from build123d import *

# Parameters (mm, degrees)
BOSS_EXTRUDE1_DEPTH = 5
SKETCH4_R           = 2.5
CUT_EXTRUDE1_DEPTH  = 20
CUT_EXTRUDE2_DEPTH  = 10
SKETCH8_R           = 2.5
CUT_EXTRUDE3_DEPTH  = 10


with BuildPart() as part:
    # Sketch1 → Boss-Extrude1 (new body)
    with BuildSketch(Plane(origin=(0, 0, 0), x_dir=(1, 0, 0), z_dir=(0, 1, 0))):
        with BuildLine():
            Line((-279.827757823, 163.191662052), (-273.826637764, 163.191662052))
            ThreePointArc((-273.826637764, 163.191662052), (-271.35176403, 162.166535786), (-270.326637764, 159.691662052))
            Line((-270.326637764, 159.691662052), (-270.326637764, 137.406790352))
            Line((-270.326637764, 137.406790352), (-275.326637764, 137.406790352))
            Line((-275.326637764, 137.406790352), (-275.326637764, -155.644744292))
            Line((-275.326637764, -155.644744292), (-270.326637764, -155.644744292))
            Line((-270.326637764, -155.644744292), (-270.326637764, -177.929615992))
            ThreePointArc((-270.326637764, -177.929615992), (-271.35176403, -180.404489727), (-273.826637764, -181.429615992))
            Line((-273.826637764, -181.429615992), (-279.827757823, -181.429615992))
            ThreePointArc((-279.827757823, -181.429615992), (-293.34742446, -188.470830973), (-295.328317853, -203.584935503))
            ThreePointArc((-295.328317853, -203.584935503), (-279.434102169, -225.521844766), (-254.372898367, -235.807278357))
            ThreePointArc((-254.372898367, -235.807278357), (-245.944078079, -233.964230965), (-239.597831877, -228.11897697))
            Line((-239.597831877, -228.11897697), (-235.326637764, -228.11897697))
            Line((-235.326637764, -228.11897697), (-235.326637764, -233.11897697))
            Line((-235.326637764, -233.11897697), (161.673362236, -233.11897697))
            Line((161.673362236, -233.11897697), (161.673362236, -228.11897697))
            Line((161.673362236, -228.11897697), (165.944556349, -228.11897697))
            ThreePointArc((165.944556349, -228.11897697), (172.290802551, -233.964230965), (180.719622838, -235.807278357))
            ThreePointArc((180.719622838, -235.807278357), (205.780826641, -225.521844766), (221.675042324, -203.584935503))
            ThreePointArc((221.675042324, -203.584935503), (219.694148932, -188.470830973), (206.174482295, -181.429615992))
            Line((206.174482295, -181.429615992), (200.173362236, -181.429615992))
            ThreePointArc((200.173362236, -181.429615992), (197.698488502, -180.404489727), (196.673362236, -177.929615992))
            Line((196.673362236, -177.929615992), (196.673362236, -155.644744292))
            Line((196.673362236, -155.644744292), (201.673362236, -155.644744292))
            Line((201.673362236, -155.644744292), (201.673362236, 137.406790352))
            Line((201.673362236, 137.406790352), (196.673362236, 137.406790352))
            Line((196.673362236, 137.406790352), (196.673362236, 159.691662052))
            ThreePointArc((196.673362236, 159.691662052), (197.698488502, 162.166535786), (200.173362236, 163.191662052))
            Line((200.173362236, 163.191662052), (206.174482295, 163.191662052))
            ThreePointArc((206.174482295, 163.191662052), (219.694148932, 170.232877033), (221.675042324, 185.346981563))
            ThreePointArc((221.675042324, 185.346981563), (205.780826641, 207.283890825), (180.719622838, 217.569324417))
            ThreePointArc((180.719622838, 217.569324417), (172.290802551, 215.726277025), (165.944556349, 209.88102303))
            Line((165.944556349, 209.88102303), (161.673362236, 209.88102303))
            Line((161.673362236, 209.88102303), (161.673362236, 214.88102303))
            Line((161.673362236, 214.88102303), (-235.326637764, 214.88102303))
            Line((-235.326637764, 214.88102303), (-235.326637764, 209.88102303))
            Line((-235.326637764, 209.88102303), (-239.597831877, 209.88102303))
            ThreePointArc((-239.597831877, 209.88102303), (-245.944078079, 215.726277025), (-254.372898367, 217.569324417))
            ThreePointArc((-254.372898367, 217.569324417), (-279.434102169, 207.283890825), (-295.328317853, 185.346981563))
            ThreePointArc((-295.328317853, 185.346981563), (-293.34742446, 170.232877033), (-279.827757823, 163.191662052))
        make_face()
    extrude(amount=BOSS_EXTRUDE1_DEPTH)

    # Sketch4 → Cut-Extrude1 (cut)
    with BuildSketch(Plane.XZ):
        with Locations(Location((-201.826637764, 124.11897697, 0), (0, 0, 270))):
            Circle(SKETCH4_R)
        with Locations(Location((-201.826637764, -105.88102303, 0), (0, 0, 90))):
            Circle(SKETCH4_R)
        with Locations(Location((128.173362236, -105.88102303, 0), (0, 0, 270))):
            Circle(SKETCH4_R)
        with Locations(Location((128.173362236, 124.11897697, 0), (0, 0, 90))):
            Circle(SKETCH4_R)
    extrude(amount=-CUT_EXTRUDE1_DEPTH, mode=Mode.SUBTRACT)

    # Sketch5 → Cut-Extrude2 (cut)
    with BuildSketch(Plane(origin=(0, 5, 0), x_dir=(1, 0, 0), z_dir=(0, 1, 0))):
        with BuildLine():
            Line((-255.326637764, -44.11897697), (-255.326637764, 25.88102303))
            ThreePointArc((-255.326637764, 25.88102303), (-235.326637764, 45.88102303), (-215.326637764, 25.88102303))
            Line((-215.326637764, 25.88102303), (-215.326637764, -44.11897697))
            ThreePointArc((-215.326637764, -44.11897697), (-235.326637764, -64.11897697), (-255.326637764, -44.11897697))
        make_face()
    extrude(amount=-CUT_EXTRUDE2_DEPTH, mode=Mode.SUBTRACT)

    # Sketch8 → Cut-Extrude3 (cut)
    with BuildSketch(Plane.XZ):
        with Locations(Location((-201.826637764, -105.88102303, 0), (0, 0, 90))):
            Circle(SKETCH8_R)
        with Locations(Location((-201.826637764, -5.88102303, 0), (0, 0, 270))):
            Circle(SKETCH8_R)
        with Locations(Location((-12.826637764, -5.88102303, 0), (0, 0, 270))):
            Circle(SKETCH8_R)
        with Locations(Location((-12.826637764, -105.88102303, 0), (0, 0, 270))):
            Circle(SKETCH8_R)
    extrude(amount=-CUT_EXTRUDE3_DEPTH, mode=Mode.SUBTRACT)


solid = part.part
Design review of the part built by this model. Coordinates are the model's own, in mm. A direction names the side the tool comes from. Give positions to 0.01 mm unless a question says otherwise; leave off trailing zeros. Write each loop counter-clockwise with the first axis right and the second up, starting at its lowest first coordinate (ties: lowest second). Pieces come first, ordered by that corner, then holes. Notation, with made-up numbers: M 55,31 L 70,31 A24 ccw 70,56 Z; hole C -20.5,-16 d9. An arc over 180 degrees is marked long. Return JSON: item names as keys, results as strings. Group by question number.
Item 1: Tool access review of faces 1 (the cylindrical face through (-293.473, 2.465, -170.415)), 2 (the cylindrical face through (-234.887, 2.535, 64.114)): name each direction out of +Z, -Z, +X, -X, +Y, -Y from which nothing blocks a thin tool from reaching the whole face with its end or side.
Item 2: Wall thickness on line 1 along Z through (x, y) = (-202.5, 3.5); line 2 along Z through (x, y) = (129, 3.15); line 3 along Z through (x, y) = (-200, 1.2): over which ranges is each line inside the solid? List them lowest first.
Item 3: Take a section at C-C (y = 2). Count the separate pieces of the cut face and the enclosed holes in it, plus the area to 3 significant figures.
Item 4: Take a section at B-B (z = -150.5). Give the boundary of the cut face in (x, y), plus the area to 4 significant figures.
Item 5: The part is to be moulded in two halves that separate along Z. For faces 3 (the cylindrical face through (-293.22, 2.46, 188.29)), 4 (the cylindrical face through (-235.766, 2.535, -45.876)), 5 (the flat face through (-40, 5, 6)), 6 (the cylindrical face through (205.478, 2.465, 225.758)), say which applies: pulls with the +Z half, pulls with the -Z half, needs draft (parallel to the pull), parting line crosses it, or undercut.
Item 6: Take a section at A-A (x = -227). Give the boundary of the cut face in (y, z).
Item 7: Clearance check with flat-ended pins moving along their axes: pin 1 Ø1.5 at (x, y) = (-6, 2) entering from +Z; pin 2 Ø2 at (x, y) = (164.5, 3.5) entering from -Z; pin 3 Ø2 at (y, z) = (1.5, -105.5) entering from +X; pin 4 Ø4.5 at (x, z) = (128.17, -105.88) entering from -Y. State where each tip first meets the part, or that it passes through.
Return value:
{
 "1": {"face 1": "-X, +Y, -Y", "face 2": "+Y, -Y"},
 "2": {"line 1": "z = -214.88 to -108.29, -103.47 to -8.29, -3.47 to 121.71, 126.53 to 233.12", "line 2": "z = -214.88 to -108.24, -103.52 to 121.76, 126.48 to 233.12", "line 3": "z = -214.88 to -107.59, -104.17 to -7.59, -4.17 to 122.41, 125.83 to 233.12"},
 "3": {"separate pieces": "1", "enclosed holes": "8", "area": "212,000 mm2"},
 "4": {"outline": "M -270.33,0 L 196.67,0 L 196.67,5 L -270.33,5 Z", "area": "2,335 mm2"},
 "5": {"face 3": "undercut", "face 4": "undercut", "face 5": "needs draft", "face 6": "pulls with the +Z half"},
 "6": {"outline": "M 0,-214.88 L 5,-214.88 L 5,-44.07 L 0,-44.07 Z; M 0,62.3 L 5,62.3 L 5,233.12 L 0,233.12 Z"},
 "7": {"pin 1": "stops at z = 233.12", "pin 2": "stops at z = -209.88", "pin 3": "stops at x = 201.67", "pin 4": "passes through"}
}
